```python
from build123d import *

# Parameters (mm, degrees)
SKETCH3_W           = 25
SKETCH3_H           = 180
BOSS_EXTRUDE1_DEPTH = 25
SKETCH4_W           = 14
SKETCH4_H           = 40
CUT_EXTRUDE1_DEPTH  = 183.157212319
SKETCH6_W           = 25
SKETCH6_H           = 12.5
CUT_EXTRUDE2_DEPTH  = 183.26628871
SKETCH6_3_R         = 0.95
CUT_EXTRUDE3_DEPTH  = 9
SKETCH8_W           = 25
SKETCH8_H           = 12.5
CUT_EXTRUDE4_DEPTH  = 183.26628871
SKETCH8_3_R         = 0.95
CUT_EXTRUDE5_DEPTH  = 9
FILLET1_R           = 4
CUT_EXTRUDE6_START  = -2
SKETCH12_W          = 3.466571871
SKETCH12_H          = 5
CUT_EXTRUDE6_DEPTH  = 10
CUT_EXTRUDE7_START  = -2
SKETCH11_W          = 3.979632528
SKETCH11_H          = 5
CUT_EXTRUDE7_DEPTH  = 14
FILLET2_R           = 4
FILLET3_R           = 4


with BuildPart() as part:
    # Sketch3 → Boss-Extrude1 (new body)
    with BuildSketch(Plane(origin=(0, 0, 0), x_dir=(1, 0, 0), z_dir=(0, 1, 0))):
        with Locations((0, 90)):
            Rectangle(SKETCH3_W, SKETCH3_H)
    extrude(amount=BOSS_EXTRUDE1_DEPTH)

    # Sketch4 → Cut-Extrude1 (cut, through all)
    with BuildSketch(Plane(origin=(0, 25, 0), x_dir=(1, 0, 0), z_dir=(0, 1, 0))):
        with Locations((5.5, 160)):
            Rectangle(SKETCH4_W, SKETCH4_H)
        with Locations((-5.5, 20)):
            Rectangle(SKETCH4_W, SKETCH4_H)
    extrude(amount=-CUT_EXTRUDE1_DEPTH, mode=Mode.SUBTRACT)

    # Sketch6 → Cut-Extrude2 (cut, through all)
    with BuildSketch(Plane.ZY.offset(-1.5)):
        with Locations((-18.82, 12.5)):
            Rectangle(SKETCH6_W, SKETCH6_H)
    extrude(amount=-CUT_EXTRUDE2_DEPTH, mode=Mode.SUBTRACT)

    # Sketch6_3 → Cut-Extrude3 (cut)
    with BuildSketch(Plane.ZY.offset(-1.5)):
        with Locations((-32.57, 12.5)):
            Circle(SKETCH6_3_R)
        with Locations((-5.07, 12.5)):
            Circle(SKETCH6_3_R)
    extrude(amount=-CUT_EXTRUDE3_DEPTH, mode=Mode.SUBTRACT)

    # Sketch8 → Cut-Extrude4 (cut, through all)
    with BuildSketch(Plane(origin=(-1.5, 0, 0), x_dir=(0, 0, -1), z_dir=(1, 0, 0))):
        with Locations((161.18, 12.5)):
            Rectangle(SKETCH8_W, SKETCH8_H)
    extrude(amount=-CUT_EXTRUDE4_DEPTH, mode=Mode.SUBTRACT)

    # Sketch8_3 → Cut-Extrude5 (cut)
    with BuildSketch(Plane(origin=(-1.5, 0, 0), x_dir=(0, 0, -1), z_dir=(1, 0, 0))):
        with Locations((147.43, 12.5)):
            Circle(SKETCH8_3_R)
        with Locations(Location((174.93, 12.5, 0), (0, 0, 180))):
            Circle(SKETCH8_3_R)
    extrude(amount=-CUT_EXTRUDE5_DEPTH, mode=Mode.SUBTRACT)

    # Fillet1
    fillet1_edges = [part.edges().sort_by_distance(p)[0] for p in [
        (-12.5, 0, -110),
        (-12.5, 25, -110),
        (12.5, 0, -70),
        (12.5, 25, -70),
    ]]
    fillet(fillet1_edges, radius=FILLET1_R)

    # Sketch12 → Cut-Extrude6 (cut)
    with BuildSketch(Plane(origin=(-1.5, 0, 0), x_dir=(0, 0, -1), z_dir=(1, 0, 0)).offset(CUT_EXTRUDE6_START)):
        with Locations((146.946714065, 12.5)):
            Rectangle(SKETCH12_W, SKETCH12_H)
    extrude(amount=-CUT_EXTRUDE6_DEPTH, mode=Mode.SUBTRACT)

    # Sketch11 → Cut-Extrude7 (cut)
    with BuildSketch(Plane.ZY.offset(-1.5).offset(CUT_EXTRUDE7_START)):
        with Locations((-33.309816264, 12.5)):
            Rectangle(SKETCH11_W, SKETCH11_H)
    extrude(amount=-CUT_EXTRUDE7_DEPTH, mode=Mode.SUBTRACT)

    # Fillet2
    fillet2_edges = [part.edges().sort_by_distance(p)[0] for p in [
        (-5, 0, -180),
        (-12.5, 12.5, -180),
        (-5, 25, -180),
        (-11.328427125, 23.828427125, -180),
        (-11.328427125, 1.171572875, -180),
    ]]
    fillet(fillet2_edges, radius=FILLET2_R)

    # Fillet3
    fillet3_edges = [part.edges().sort_by_distance(p)[0] for p in [
        (12.5, 12.5, 0),
        (11.328427125, 23.828427125, 0),
        (11.328427125, 1.171572875, 0),
        (5, 0, 0),
        (5, 25, 0),
    ]]
    fillet(fillet3_edges, radius=FILLET3_R)


solid = part.part
```
The listing builds one solid part. Answer for the finished solid, in the listing's coordinates (mm). A direction names the side the tool comes from. Coordinates: 2 decimals unless noted, no trailing zeros. Loops run counter-clockwise (first coordinate to the right, second up) from the corner with the lowest first, then second, coordinate; pieces in that order, holes last. Notation, with made-up numbers: (43, -20) - (68, -20) arc R34 ccw to (68, 10) - close; hole circle Ø7 at (10.5, -25.5). An arc over 180 degrees is marked (long way). Use a Markdown table: item, result. Add a question column.
1) The part is cut by section A-A, the plane z = -166. Give the vertices of the cut face in (x, y), and give its area (3 significant figures).
2) Find the intervals of material crossed by line 1 (Z direction, x = -6.75, y = 12.5); line 2 (Y direction, x = -8, z = -174.93); line 3 (Z direction, x = 9, y = 19.5), in increasing order.
3) Given pin 1 (12 mm diameter, centred on x = 4, y = 12.5, fed in from -Z); pin 2 (3.5 mm diameter, centred on x = -7, y = 14.5, fed in from +Z); pin 3 (5.5 mm diameter, centred on x = 6.5, y = 10.5, fed in from -Z); pin 4 (1 mm diameter, centred on y = 13, z = -147.5, fed in from -X), each flat-ended and moving along its own axis, determine where each tip first touches the part or whether it passes through.
4) The part is cut by section B-B, the plane x = 5.25. Give the vertices of the cut face in (y, z), and give its area (3 significant figures).
5) For faces 5 (the flat face through (8, 12, -35.3)), 6 (the flat face through (-8, 12, -145.213)), 7 (the flat face through (7, 18.75, -19)), determine the directions among +Z, -Z, +X, -X, +Y, -Y from which every point of the face is accessible in a straight line to the end or side of a thin tool.
6) The mould has two halves that part along Z. Classify faces 1 (the flat face through (0, 0, -91)), 2 (the flat face through (8, 10, -33)), 3 (the flat face through (5, 13, -140)), 4 (the flat face through (5, 12, 0)): released by +Z, released by -Z, zero draft, split by the parting line, or undercut.
Here are the results:
| question | item | result |
|---|---|---|
| 1 | outline | (-12.5, 4) arc R4 ccw to (-8.5, 0) - (-1.5, 0) - (-1.5, 6.25) - (-12.5, 6.25) - close; (-12.5, 18.75) - (-1.5, 18.75) - (-1.5, 25) - (-8.5, 25) arc R4 ccw to (-12.5, 21) - close |
| 1 | area | 131 mm^2 |
| 2 | line 1 | z = -180 to -175.88, -173.98 to -173.68, -145.21 to -40 |
| 2 | line 2 | y = 0 to 11.55, 13.45 to 25 |
| 2 | line 3 | z = -140 to -0.03 |
| 3 | pin 1 | stops at z = -180 |
| 3 | pin 2 | stops at z = -40 |
| 3 | pin 3 | stops at z = -140 |
| 3 | pin 4 | stops at x = -3.5 |
| 4 | outline | (0, -140) - (25, -140) - (25, -4) arc R4 ccw to (21, 0) - (4, 0) arc R4 ccw to (0, -4) - close; hole (6.25, -31.32) - (10, -31.32) - (10, -35.3) - (15, -35.3) - (15, -31.32) - (18.75, -31.32) - (18.75, -6.32) - (6.25, -6.32) - close; hole circle Ø1.9 at (12.5, -5.07) |
| 4 | area | 3,160 mm^2 |
| 5 | face 5 | +X |
| 5 | face 6 | -X |
| 5 | face 7 | +X, -X |
| 6 | face 1 | zero draft |
| 6 | face 2 | undercut |
| 6 | face 3 | released by -Z |
| 6 | face 4 | released by +Z |
